```python
from build123d import *

# Parameters (mm, degrees)
SKETCH1_R           = 3.75
BOSS_EXTRUDE1_DEPTH = 15
SKETCH2_R           = 20
BOSS_EXTRUDE2_DEPTH = 20
SKETCH4_R           = 10
CUT_EXTRUDE1_DEPTH  = 35


with BuildPart() as part:
    # Sketch1 → Boss-Extrude1 (new body)
    with BuildSketch(Plane.XY):
        with BuildLine():
            Line((45, 55), (85, 55))
            ThreePointArc((85, 55), (100, 40), (85, 25))
            Line((85, 25), (73.301270189, 25))
            ThreePointArc((73.301270189, 25), (53.864269805, 21.067374747), (37.484806964, 9.888120643))
            ThreePointArc((37.484806964, 9.888120643), (32.346878, 2.774072366), (29.48734245, -5.522375871))
            ThreePointArc((29.48734245, -5.522375871), (-1.978417772, -29.934693303), (-29.957644649, -1.593589371))
            ThreePointArc((-29.957644649, -1.593589371), (-29.930461106, -0.154464501), (-29.696951333, 1.265849732))
            Line((-29.696951333, 1.265849732), (-19.587782351, 43.492363969))
            ThreePointArc((-19.587782351, 43.492363969), (-14.290170624, 51.776787753), (-5, 55))
            Line((-5, 55), (45, 55))
        make_face()
        with Locations((-5, 40)):
            Circle(SKETCH1_R, mode=Mode.SUBTRACT)
        with BuildLine():
            Line((45, 46), (85, 46))
            ThreePointArc((85, 46), (91, 40), (85, 34))
            Line((85, 34), (45, 34))
            ThreePointArc((45, 34), (39, 40), (45, 46))
        make_face(mode=Mode.SUBTRACT)
    extrude(amount=BOSS_EXTRUDE1_DEPTH)

    # Sketch2 → Boss-Extrude2 (add)
    with BuildSketch(Plane.XY.offset(15)):
        Circle(SKETCH2_R)
    extrude(amount=BOSS_EXTRUDE2_DEPTH)

    # Sketch4 → Cut-Extrude1 (cut)
    with BuildSketch(Plane.XY.offset(35)):
        Circle(SKETCH4_R)
    extrude(amount=-CUT_EXTRUDE1_DEPTH, mode=Mode.SUBTRACT)


solid = part.part
```
Design review of the part built by this model. Coordinates are the model's own, in mm. A direction names the side the tool comes from. Coordinates: 2 decimals unless noted, no trailing zeros. Order: outer loops, then holes, each group sorted by start corner. A loop starts at its lowest first (then second) coordinate and runs counter-clockwise, first axis right, second up. Notation, with made-up numbers: M -10.5,39 L -1.5,39 A14 cw -1.5,55 Z; hole C 23.5,9.25 d6. An arc over 180 degrees is marked long. Answer as a JSON object with one key per item and string values. Group by question number.
1) Add section A-A, the plane x = 75.5. Write out the cut boundary in (y, z), then the cut area to 3 significant figures.
2) For pin 1 (6 mm diameter, centred on x = 4, y = -12, fed in from -Z); pin 2 (2 mm diameter, centred on x = 43.5, z = 15.5, fed in from -Y); pin 3 (13 mm diameter, centred on x = 77, z = 10, fed in from -Y); pin 4 (10 mm diameter, centred on x = 32.5, y = 13.5, fed in from +Z), all flat-tipped, find the tip position at first contact; note any pin that passes through.
3) Mouldability with a two-part tool opening along Y and no side actions: class faces 4 (the flat face through (79, 25, 7)), 5 (the cylindrical face through (100, 40, 7)), 6 (the cylindrical face through (-14, 52, 7)), 7 (the cylindrical face through (-5.81, 36.34, 7.4)) as pulls with the +Y half, pulls with the -Y half, needs draft (parallel to the pull), parting line crosses it, or undercut.
4) Tool access review of faces 1 (the flat face through (65, 34, 7)), 2 (the cylindrical face through (-4.336, -19.524, 24.86)), 3 (the flat face through (-5, 9, 35)): name each direction out of +Z, -Z, +X, -X, +Y, -Y from which nothing blocks a thin tool from reaching the whole face with its end or side.
5) Wall thickness on L1, parallel to X at y = 0.5, z = 17; L2, parallel to Y at x = 0, z = 8; L3, parallel to Z at x = 19.5, y = -13: over which ranges is each line inside the solid? List them lowest first.
6) Add section B-B, the plane z = 11.5. Write out the cut boundary in (x, y), then the cut area to 3 significant figures.
7) Add section D-D, the plane z = 30. Write out the cut boundary in (x, y).
8) Add section C-C, the plane y = 3. Write out the cut boundary in (x, z), then the cut area to 3 significant figures.
Computed values:
{
 "1": {"outline": "M 25,0 L 34,0 L 34,15 L 25,15 Z; M 46,0 L 55,0 L 55,15 L 46,15 Z", "area": "270 mm^2"},
 "2": {"pin 1": "stops at z = 0", "pin 2": "stops at y = 14.49", "pin 3": "stops at y = 24.92", "pin 4": "stops at z = 15"},
 "3": {"face 4": "pulls with the -Y half", "face 5": "parting line crosses it", "face 6": "pulls with the +Y half", "face 7": "undercut"},
 "4": {"face 1": "+Z, -Z", "face 2": "+Z", "face 3": "+Z, +X, -X, +Y, -Y"},
 "5": {"L1": "x = -19.99 to -9.99, 9.99 to 19.99", "L2": "y = -30 to -10, 10 to 55", "L3": "z = 0 to 15"},
 "6": {"outline": "M -29.96,-1.59 A30 ccw 29.49,-5.52 A30 cw 37.48,9.89 A50 cw 73.3,25 L 85,25 A15 ccw 85,55 L -5,55 A15 ccw -19.59,43.49 L -29.7,1.27 A10 ccw Z; hole C 0,0 d20; hole C -5,40 d7.5; hole M 45,34 L 85,34 A6 ccw 85,46 L 45,46 A6 ccw Z", "area": "5,700 mm^2"},
 "7": {"outline": "C 0,0 d40; hole C 0,0 d20"},
 "8": {"outline": "M -29.28,0 L -9.54,0 L -9.54,35 L -19.77,35 L -19.77,15 L -29.28,15 Z; M 9.54,0 L 32.47,0 L 32.47,15 L 19.77,15 L 19.77,35 L 9.54,35 Z", "area": "1,050 mm^2"}
}
